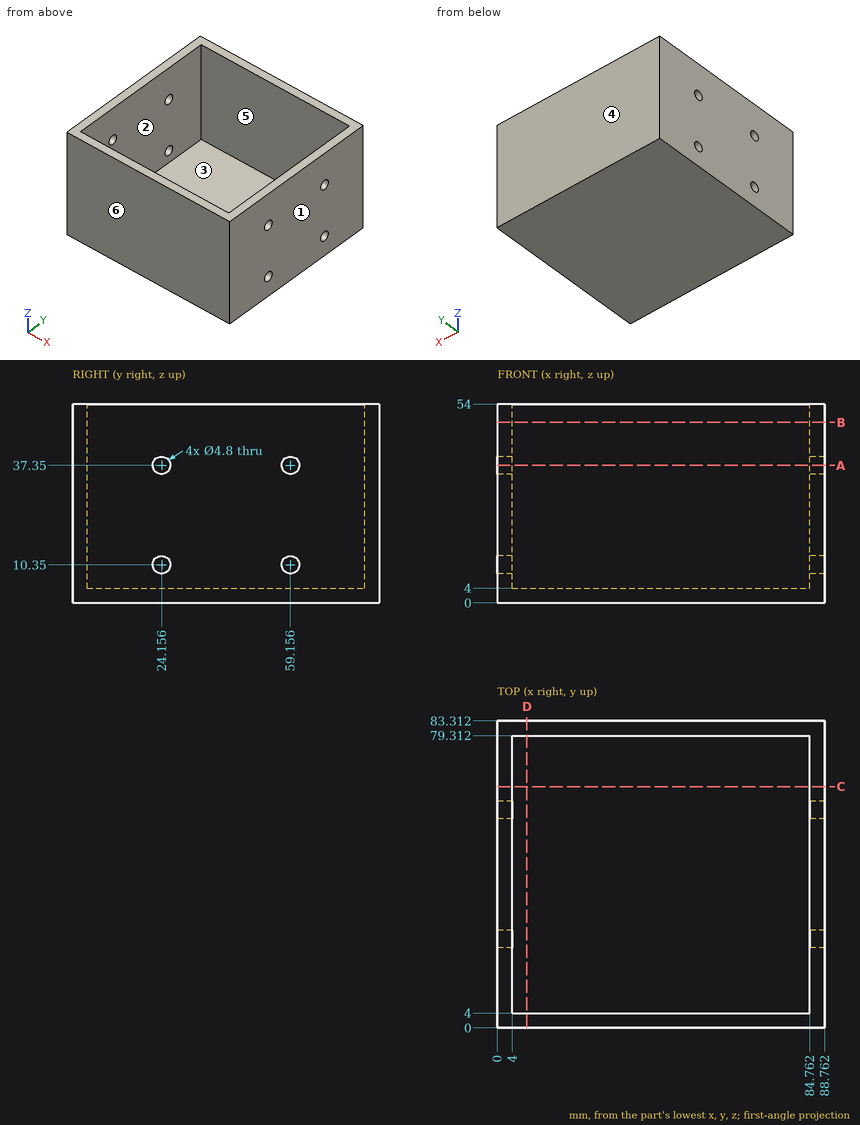
Job drawing, mm, ordinate dimensions from the low corner. One solid piece. A direction names the side the tool comes from. Give positions to 0.01 mm unless a question says otherwise; leave off trailing zeros. Write each loop counter-clockwise with the first axis right and the second up, starting at its lowest first coordinate (ties: lowest second). Pieces come first, ordered by that corner, then holes. Notation, with made-up numbers: M 14.25,29 L 31.25,29 A27 cw 31.25,52 Z; hole C 3.25,-0.75 d11. An arc over 180 degrees is marked long. One line per item, written item: value. Start each with the question number.
Q1. Probe probe 1 along Y at (x, z) = (87, 10); probe 2 along Y at (x, z) = (86, 37.35); probe 3 along X at (y, z) = (31.5, 25). List the from-to ranges inside material, lowest first. Write a range as [from, to].
Q2. 3-axis set-ups, long thin cutter, end or side, ignore diameter. For the marked faces 5 and 6: which of +Z, -Z, +X, -X, +Y, -Y reach the whole face in a straight line?
Q3. Saw through at D-D, the plane x = 8. Write the cut outline in (y, z).
Q4. Saw through at C-C, the plane y = 65.5. Write the cut outline in (x, z).
Q5. Two-plate mould, pull along X, no slides. Class the marked faces 1, 2, 3 and 4: +X half, -X half, draft (parallel to the pull), parting line (faces both ways), or undercut.
Q6. Drop flat-ended pins along their axis: pin 1 Ø10 at (y, z) = (49.5, 22.5) entering from -X; pin 2 Ø8 at (x, y) = (53.5, 45.5) entering from +Z. Give the stop position or say it passes through.
Q7. Saw through at B-B, the plane z = 49. Write the cut outline in (x, y).
Q8. Saw through at A-A, the plane z = 37.35. Write the cut outline in (x, y), plus the area to 3 significant figures.
Output values:
1. probe 1: y = [0, 21.78], [26.53, 56.78], [61.53, 83.31]
1. probe 2: y = [0, 21.76], [26.56, 56.76], [61.56, 83.31]
1. probe 3: x = [0, 4], [84.76, 88.76]
2. face 5: +Z
2. face 6: +Z, -Z, +X, -X, -Y
3. outline: M 0,0 L 83.31,0 L 83.31,54 L 79.31,54 L 79.31,4 L 4,4 L 4,54 L 0,54 Z
4. outline: M 0,0 L 88.76,0 L 88.76,54 L 84.76,54 L 84.76,4 L 4,4 L 4,54 L 0,54 Z
5. face 1: +X half
5. face 2: undercut
5. face 3: undercut
5. face 4: draft
6. pin 1: stops at x = 0
6. pin 2: stops at z = 4
7. outline: M 0,0 L 88.76,0 L 88.76,83.31 L 0,83.31 Z; hole M 4,4 L 84.76,4 L 84.76,79.31 L 4,79.31 Z
8. outline: M 0,0 L 88.76,0 L 88.76,21.76 L 84.76,21.76 L 84.76,4 L 4,4 L 4,21.76 L 0,21.76 Z; M 0,26.56 L 4,26.56 L 4,56.76 L 0,56.76 Z; M 0,61.56 L 4,61.56 L 4,79.31 L 84.76,79.31 L 84.76,61.56 L 88.76,61.56 L 88.76,83.31 L 0,83.31 Z; M 84.76,26.56 L 88.76,26.56 L 88.76,56.76 L 84.76,56.76 Z
8. area: 1,240 mm²
